```python
from build123d import *

# Parameters (mm, degrees)
SKETCH1_W                      = 8
SKETCH1_H                      = 50
BOSS_EXTRUDE1_DEPTH            = 6
SKETCH2_W                      = 8
SKETCH2_H                      = 10
CUT_EXTRUDE2_DEPTH             = 5
CUT_EXTRUDE3_REACH             = 28.019
SKETCH3_R                      = 2
FILLET1_R                      = 3
FILLET2_R                      = 7
SKETCH4_W                      = 8
SKETCH4_H                      = 8
BOSS_EXTRUDE2_DEPTH            = 15
CUT_EXTRUDE4_REACH             = 34.894
CUT_EXTRUDE4_DIRECTION_2_DEPTH = 33.893768419


with BuildPart() as part:
    # Sketch1 → Boss-Extrude1 (new body)
    with BuildSketch(Plane(origin=(0, 0, 0), x_dir=(1, 0, 0), z_dir=(0, 1, 0))):
        Rectangle(SKETCH1_W, SKETCH1_H)
    extrude(amount=BOSS_EXTRUDE1_DEPTH)

    # Sketch2 → Cut-Extrude2 (cut)
    with BuildSketch(Plane.XZ):
        with Locations((0, 20)):
            Rectangle(SKETCH2_W, SKETCH2_H)
    extrude(amount=-CUT_EXTRUDE2_DEPTH, mode=Mode.SUBTRACT)

    # Sketch3 → Cut-Extrude3 (cut, up to next)
    with BuildSketch(Plane(origin=(0, 6, 0), x_dir=(1, 0, 0), z_dir=(0, 1, 0)), mode=Mode.PRIVATE) as cut_extrude3_sk1:
        with Locations(Location((0, -22, 0), (0, 0, 270))):
            Circle(SKETCH3_R)
    cut_extrude3_tool1 = extrude(cut_extrude3_sk1.sketch, amount=-CUT_EXTRUDE3_REACH, mode=Mode.PRIVATE) & part.part
    add(cut_extrude3_tool1.solids().sort_by_distance((0, 6, 22))[0], mode=Mode.SUBTRACT)

    # Fillet1
    fillet1_edges = [part.edges().sort_by_distance(p)[0] for p in [
        (4, 5.5, 25),
        (-4, 5.5, 25),
    ]]
    fillet(fillet1_edges, radius=FILLET1_R)

    # Fillet2
    # the kernel refuses this fillet: 7 mm, written as the material it adds along each edge
    with BuildSketch(Plane(origin=(-4, 5, 15), x_dir=(0, 0, 1), z_dir=(1, 0, 0))) as fillet2_piece_1_section:
        with BuildLine():
            CenterArc((6.708203932, 7), FILLET2_R, 196.601549599, 73.398450401)
            Line((0, 5), (0, 0))
            Line((0, 0), (6.708203932, 0))
        make_face()
    fillet2_piece_1 = extrude(amount=8, mode=Mode.PRIVATE)
    fillet2_piece_1 = fillet2_piece_1 - Plane(origin=(0, 5, 22), x_dir=(0, 0, 1), z_dir=(0, 1, 0)) * Cylinder(2, 43, mode=Mode.PRIVATE)
    add(fillet2_piece_1)

    # Sketch4 → Boss-Extrude2 (add)
    with BuildSketch(Plane(origin=(0, 0, 0), x_dir=(-1, 0, 0), z_dir=(0, -1, 0))):
        with Locations((0, 21)):
            Rectangle(SKETCH4_W, SKETCH4_H)
    extrude(amount=BOSS_EXTRUDE2_DEPTH)

    # Sketch5 → Cut-Extrude4 (cut, up to next)
    with BuildSketch(Plane(origin=(0, 6, 0), x_dir=(1, 0, 0), z_dir=(0, 1, 0)), mode=Mode.PRIVATE) as cut_extrude4_sk1:
        Polygon((4, 25), (4, 23), (2, 23), align=None)
    cut_extrude4_tool1 = extrude(cut_extrude4_sk1.sketch, amount=-CUT_EXTRUDE4_REACH, mode=Mode.PRIVATE) & part.part
    # Sketch5 → Cut-Extrude4 (cut, up to next)
    with BuildSketch(Plane(origin=(0, 6, 0), x_dir=(1, 0, 0), z_dir=(0, 1, 0)), mode=Mode.PRIVATE) as cut_extrude4_sk2:
        Polygon((-4, 25), (-4, 23), (-2, 23), align=None)
    cut_extrude4_tool2 = extrude(cut_extrude4_sk2.sketch, amount=-CUT_EXTRUDE4_REACH, mode=Mode.PRIVATE) & part.part
    add(cut_extrude4_tool1.solids().sort_by_distance((3.333333, 6, -23.666667))[0], mode=Mode.SUBTRACT)
    add(cut_extrude4_tool2.solids().sort_by_distance((-3.333333, 6, -23.666667))[0], mode=Mode.SUBTRACT)

    # Sketch5 → Cut-Extrude4 direction 2 (cut)
    with BuildSketch(Plane(origin=(0, 6, 0), x_dir=(1, 0, 0), z_dir=(0, 1, 0))):
        Polygon((4, 25), (4, 23), (2, 23), align=None)
        Polygon((-4, 25), (-4, 23), (-2, 23), align=None)
    extrude(amount=CUT_EXTRUDE4_DIRECTION_2_DEPTH, mode=Mode.SUBTRACT)


solid = part.part
```
Input: part model. Units: mm. Frame: model coordinates. A direction names the side the tool comes from. Coordinates: 2 decimals unless noted, no trailing zeros. Write each loop counter-clockwise with the first axis right and the second up, starting at its lowest first coordinate (ties: lowest second). Pieces come first, ordered by that corner, then holes. Notation, with made-up numbers: (69, 53) -> (116, 53) arc R18 cw to (116, 74) -> close; hole circle Ø6 at (77, 1.25). An arc over 180 degrees is marked (long way). Write each question's results on one line, items separated by ' | '.
Item 1: Set-up query: faces 5 (the flat face through (0, -7, -17)), 6 (the cylindrical face through (0.088, 5.537, 20.002)). Return all of +Z, -Z, +X, -X, +Y, -Y with unobstructed straight access to the full face (end or side cutting, diameter ignored); none if empty.
Conclusion:
face 5: +Z, +X, -X, -Y | face 6: +Y, -Y
Item 2: Section query B-B on y = -3.5. Return loops of the section in (x, z), plus the area to 3 significant figures.
Conclusion:
outline: (-4, -25) -> (4, -25) -> (2, -23) -> (4, -23) -> (4, -17) -> (-4, -17) -> (-4, -23) -> (-2, -23) -> close | area: 60.0 mm^2
Item 3: Material intervals for probe 1 along Z at (x, y) = (0, 5.1); probe 2 along X at (y, z) = (5.3, 22); probe 3 along Z at (x, y) = (-1.5, -7.5), sorted ascending.
Conclusion:
probe 1: z = -25 to 20, 24 to 25 | probe 2: x = -4 to -2, 2 to 4 | probe 3: z = -25 to -17
Item 4: Section query C-C on x = -2.5. Return loops of the section in (y, z).
Conclusion:
outline: (-15, -25) -> (6, -25) -> (6, -23.5) -> (-15, -23.5) -> close; (-15, -23) -> (6, -23) -> (6, 24.6) -> (5, 24.6) -> (5, 21.71) arc R7 cw to (0, 15) -> (0, -17) -> (-15, -17) -> close
Item 5: Pin query (flat end, axial travel): pin 1 Ø4 at (x, y) = (1, -11) entering from +Z; pin 2 Ø3.5 at (x, z) = (-0.5, 24) entering from -Y. Return the tip coordinate at first contact, or that it passes through.
Conclusion:
pin 1: stops at z = -17 | pin 2: stops at y = 5
Item 6: Section query A-A on x = 0. Return loops of the section in (y, z).
Conclusion:
outline: (-15, -25) -> (6, -25) -> (6, 20) -> (4.79, 20) arc R7 cw to (0, 15) -> (0, -17) -> (-15, -17) -> close; (5, 24) -> (6, 24) -> (6, 25) -> (5, 25) -> close
Item 7: Mould query, pull axis Z, two halves, no side actions, for faces 1 (the flat face through (0, -4, -25)), 2 (the flat face through (3, -4, -23)), 3 (the flat face through (-4, 0.3, -5.2)), 4 (the cylindrical face through (-0.06, 3.57, 17.47)). Classes: +Z half, -Z half, draft (parallel to the pull), parting line (faces both ways), or undercut.
Conclusion:
face 1: -Z half | face 2: undercut | face 3: draft | face 4: +Z half
Item 8: Section query D-D on x = 3.25. Return loops of the section in (y, z), plus the area to 3 significant figures.
Conclusion:
outline: (-15, -25) -> (6, -25) -> (6, -24.25) -> (-15, -24.25) -> close; (-15, -23) -> (6, -23) -> (6, 23.98) -> (5, 23.98) -> (5, 21.71) arc R7 cw to (0, 15) -> (0, -17) -> (-15, -17) -> close | area: 352 mm^2
